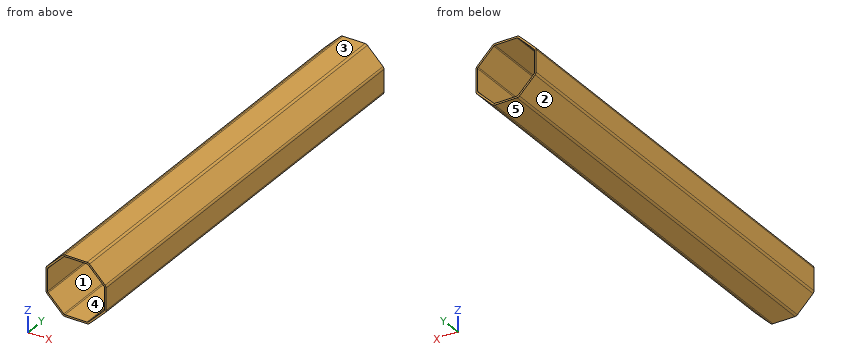
from build123d import *

# Parameters (mm, degrees)
F1_DEPTH = 500
F2_R     = 4
F3_R     = 2


with BuildPart() as f1:
    # F0 (on Front) → F1 (new body)
    with BuildSketch(Plane.XZ):
        Polygon((14.497475, 35), (-14.497475, 35), (-35, 14.497475), (-35, -14.497475), (-14.497475, -35), (14.497475, -35), (35, -14.497475), (35, 14.497475), align=None)
        Polygon((-13.669048, -33), (-33, -13.669048), (-33, 13.669048), (-13.669048, 33), (13.669048, 33), (33, 13.669048), (33, -13.669048), (13.669048, -33), align=None, mode=Mode.SUBTRACT)
    extrude(amount=F1_DEPTH)

    # F2
    f2_edges = [f1.edges().sort_by_distance(p)[0] for p in [
        (14.497475, -250, 35),
        (-14.497475, -250, 35),
        (35, -250, 14.497475),
        (35, -250, -14.497475),
        (14.497475, -250, -35),
        (-14.497475, -250, -35),
        (-35, -250, -14.497475),
        (-35, -250, 14.497475),
    ]]
    fillet(f2_edges, radius=F2_R)

    # F3
    f3_edges = [f1.edges().sort_by_distance(p)[0] for p in [
        (33, -250, 13.669048),
        (33, -250, -13.669048),
        (13.669048, -250, -33),
        (-13.669048, -250, -33),
        (-33, -250, -13.669048),
        (-33, -250, 13.669048),
        (-13.669048, -250, 33),
        (13.669048, -250, 33),
    ]]
    fillet(f3_edges, radius=F3_R)


solid = f1.part
Geometry check sheet. Reference: the model listing, model coordinates, mm. Face numbers are marked on the shaded views. A direction names the side the tool comes from. Coordinates: 2 decimals unless noted, no trailing zeros. Order: outer loops, then holes, each group sorted by start corner. A loop starts at its lowest first (then second) coordinate and runs counter-clockwise, first axis right, second up. Notation, with made-up numbers: (-4.75, 13) - (39.25, 13) arc R20 ccw to (39.25, 30) - close; hole circle Ø11 at (-25.5, 48). An arc over 180 degrees is marked (long way). Answer in a Markdown table with one row per item. Add a question column.
1) Cross-section at A-A, the plane x = -8. Record the cut outline in (y, z).
2) Gauge pin test, flat ends, axial feed: P1, Ø10, axis at y = -226.5, z = -25, coming from the +X side; P2, Ø4, axis at x = -17, y = -257, coming from the +Z side; P3, Ø10, axis at y = -90.5, z = -23, coming from the -X side. Record the tip position at first contact, or that the pin passes through.
3) Release check for a two-part mould opening along Z. For the marked faces 1, 2 and 3 record: +Z half, -Z half, draft (parallel to the pull), parting line (faces both ways), or undercut.
4) Set-up check for the marked faces 4 and 5: record each of +Z, -Z, +X, -X, +Y, -Y from which the full face is reachable in a straight line by a thin tool's end or side.
5) Material ranges on line 1 along Z through (x, y) = (-4, -367); line 2 along X through (y, z) = (-34.5, 13); line 3 along Z through (x, y) = (25, -282), recorded low to high. Write a range as [from, to].
6) Cross-section at C-C, the plane z = 6. Record the cut outline in (x, y), then the cut area to 3 significant figures.
Check result:
| question | item | result |
|---|---|---|
| 1 | outline | (-500, -35) - (0, -35) - (0, -33) - (-500, -33) - close; (-500, 33) - (0, 33) - (0, 35) - (-500, 35) - close |
| 2 | P1 | stops at x = 29.5 |
| 2 | P2 | stops at z = 34.37 |
| 2 | P3 | stops at x = -31.5 |
| 3 | face 1 | undercut |
| 3 | face 2 | -Z half |
| 3 | face 3 | +Z half |
| 4 | face 4 | +Y, -Y |
| 4 | face 5 | -Z, +X, -X, +Y, -Y |
| 5 | line 1 | z = [-35, -33], [33, 35] |
| 5 | line 2 | x = [-35, -32.99], [32.99, 35] |
| 5 | line 3 | z = [-24.5, -21.67], [21.67, 24.5] |
| 6 | outline | (-35, -500) - (-33, -500) - (-33, 0) - (-35, 0) - close; (33, -500) - (35, -500) - (35, 0) - (33, 0) - close |
| 6 | area | 2,000 mm² |
